from build123d import *

# Parameters (mm, degrees)
CROQUIS1_W              = 42.4
CROQUIS1_H              = 30.8
CROQUIS1_W_2            = 32
CROQUIS1_H_2            = 26.8
SALIENTE_EXTRUIR1_DEPTH = 6
SALIENTE_EXTRUIR2_DEPTH = 14.4
SALIENTE_EXTRUIR3_START = 2
CROQUIS1_4_W            = 42.4
CROQUIS1_4_H            = 30.8
CROQUIS1_4_W_2          = 32
CROQUIS1_4_H_2          = 26.8
CROQUIS1_4_W_3          = 2.2
CROQUIS1_4_H_3          = 2.2
SALIENTE_EXTRUIR3_DEPTH = 2
CORTAR_EXTRUIR1_REACH   = 49.353


with BuildPart() as part:
    # Croquis1 → Saliente-Extruir1 (new body)
    with BuildSketch(Plane(origin=(0, 0, 0), x_dir=(1, 0, 0), z_dir=(0, 1, 0))):
        Rectangle(CROQUIS1_W, CROQUIS1_H)
        Rectangle(CROQUIS1_W_2, CROQUIS1_H_2, mode=Mode.SUBTRACT)
    extrude(amount=-SALIENTE_EXTRUIR1_DEPTH)

    # Croquis1<3> → Saliente-Extruir2 (add)
    with BuildSketch(Plane(origin=(0, 0, 0), x_dir=(1, 0, 0), z_dir=(0, 1, 0))):
        with BuildLine():
            Line((-16, 13.4), (-16, 8.2))
            ThreePointArc((-16, 8.2), (-12.323044738, 9.723044738), (-10.8, 13.4))
            Line((-10.8, 13.4), (-16, 13.4))
        make_face()
        with BuildLine():
            Line((-16, -8.2), (-16, -13.4))
            Line((-16, -13.4), (-10.8, -13.4))
            ThreePointArc((-10.8, -13.4), (-12.323044738, -9.723044738), (-16, -8.2))
        make_face()
        with BuildLine():
            ThreePointArc((10.8, 13.4), (12.323044738, 9.723044738), (16, 8.2))
            Line((16, 8.2), (16, 13.4))
            Line((16, 13.4), (10.8, 13.4))
        make_face()
        with BuildLine():
            ThreePointArc((16, -8.2), (12.323044738, -9.723044738), (10.8, -13.4))
            Line((10.8, -13.4), (16, -13.4))
            Line((16, -13.4), (16, -8.2))
        make_face()
    extrude(amount=-SALIENTE_EXTRUIR2_DEPTH)

    # Croquis1<4> → Saliente-Extruir3 (add)
    # profile 1 of 6: a face of its own
    with BuildSketch(Plane(origin=(0, 0, 0), x_dir=(1, 0, 0), z_dir=(0, 1, 0)).offset(SALIENTE_EXTRUIR3_START)):
        Rectangle(CROQUIS1_4_W, CROQUIS1_4_H)
        Rectangle(CROQUIS1_4_W_2, CROQUIS1_4_H_2, mode=Mode.SUBTRACT)
    # profile 2 of 6: a face of its own
    with BuildSketch(Plane(origin=(0, 0, 0), x_dir=(1, 0, 0), z_dir=(0, 1, 0)).offset(SALIENTE_EXTRUIR3_START)):
        with BuildLine():
            Line((-16, -8.2), (-16, -13.4))
            Line((-16, -13.4), (-10.8, -13.4))
            ThreePointArc((-10.8, -13.4), (-12.323044738, -9.723044738), (-16, -8.2))
        make_face()
    # profile 3 of 6: a face of its own
    with BuildSketch(Plane(origin=(0, 0, 0), x_dir=(1, 0, 0), z_dir=(0, 1, 0)).offset(SALIENTE_EXTRUIR3_START)):
        with BuildLine():
            ThreePointArc((16, -8.2), (12.323044738, -9.723044738), (10.8, -13.4))
            Line((10.8, -13.4), (16, -13.4))
            Line((16, -13.4), (16, -8.2))
        make_face()
    # profile 4 of 6: a face of its own
    with BuildSketch(Plane(origin=(0, 0, 0), x_dir=(1, 0, 0), z_dir=(0, 1, 0)).offset(SALIENTE_EXTRUIR3_START)):
        with BuildLine():
            ThreePointArc((10.8, 13.4), (12.323044738, 9.723044738), (16, 8.2))
            Line((16, 8.2), (16, 13.4))
            Line((16, 13.4), (10.8, 13.4))
        make_face()
    # profile 5 of 6: a face of its own
    with BuildSketch(Plane(origin=(0, 0, 0), x_dir=(1, 0, 0), z_dir=(0, 1, 0)).offset(SALIENTE_EXTRUIR3_START)):
        with BuildLine():
            Line((-16, 13.4), (-16, 8.2))
            ThreePointArc((-16, 8.2), (-12.323044738, 9.723044738), (-10.8, 13.4))
            Line((-10.8, 13.4), (-16, 13.4))
        make_face()
    # profile 6 of 6: a face of its own
    with BuildSketch(Plane(origin=(0, 0, 0), x_dir=(1, 0, 0), z_dir=(0, 1, 0)).offset(SALIENTE_EXTRUIR3_START)):
        with BuildLine():
            ThreePointArc((-16, -8.2), (-12.323044738, -9.723044738), (-10.8, -13.4))
            Line((-10.8, -13.4), (10.8, -13.4))
            ThreePointArc((10.8, -13.4), (12.323044738, -9.723044738), (16, -8.2))
            Line((16, -8.2), (16, 8.2))
            ThreePointArc((16, 8.2), (12.323044738, 9.723044738), (10.8, 13.4))
            Line((10.8, 13.4), (3.2, 13.4))
            Line((3.2, 13.4), (3.2, 11.2))
            Line((3.2, 11.2), (1, 11.2))
            Line((1, 11.2), (1, 13.4))
            Line((1, 13.4), (-1, 13.4))
            Line((-1, 13.4), (-1, 11.2))
            Line((-1, 11.2), (-3.2, 11.2))
            Line((-3.2, 11.2), (-3.2, 13.4))
            Line((-3.2, 13.4), (-10.8, 13.4))
            ThreePointArc((-10.8, 13.4), (-12.323044738, 9.723044738), (-16, 8.2))
            Line((-16, 8.2), (-16, -8.2))
        make_face()
        with Locations((-2.1, 8.1)):
            Rectangle(CROQUIS1_4_W_3, CROQUIS1_4_H_3, mode=Mode.SUBTRACT)
        with Locations((2.1, 8.1)):
            Rectangle(CROQUIS1_4_W_3, CROQUIS1_4_H_3, mode=Mode.SUBTRACT)
    extrude(amount=-SALIENTE_EXTRUIR3_DEPTH)

    # Cortar-Extruir1: up to this face of the body (flat: up to its plane)
    cortar_extruir1_end = Plane(part.part.faces().sort_by_distance((-21.2, -2, 0))[0])
    # Croquis2 → Cortar-Extruir1 (cut, up to the picked face)
    with BuildSketch(Plane(origin=(21.2, 0, 0), x_dir=(0, 0, -1), z_dir=(1, 0, 0)), mode=Mode.PRIVATE) as cortar_extruir1_sk1:
        with BuildLine():
            Line((-2.6, -6), (2.6, -6))
            ThreePointArc((2.6, -6), (0, -3.4), (-2.6, -6))
        make_face()
    cortar_extruir1_tool1 = split(extrude(cortar_extruir1_sk1.sketch, amount=-CORTAR_EXTRUIR1_REACH, mode=Mode.PRIVATE), bisect_by=cortar_extruir1_end, keep=Keep.BOTH, mode=Mode.PRIVATE)
    add(cortar_extruir1_tool1.solids().sort_by(Axis((21.2, -4.896526, 0), (-1, 0, 0)))[0], mode=Mode.SUBTRACT)


solid = part.part
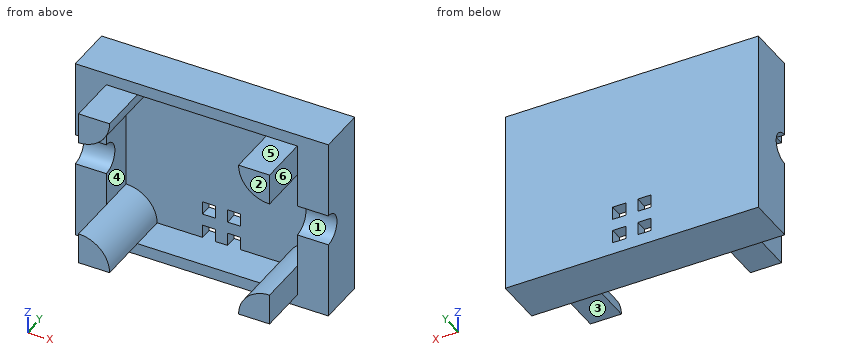
Work out the finished part from the listing and answer in its coordinate system (mm). Face numbers are marked on the shaded views. A direction names the side the tool comes from. Give positions to 0.01 mm unless a question says otherwise; leave off trailing zeros. Order: outer loops, then holes, each group sorted by start corner. A loop starts at its lowest first (then second) coordinate and runs counter-clockwise, first axis right, second up. Notation, with made-up numbers: (9.25, -7) -> (13.25, -7) arc R27 ccw to (13.25, 27) -> close; hole circle Ø5 at (9.5, -12.5). An arc over 180 degrees is marked (long way). Answer as a JSON object with one key per item and string values. Group by question number.
1. Section C-C on y = -12 is taken. Determine the outline of the cut face in (x, z).
2. The mould has two halves that part along Z. Classify the marked faces 1, 2 and 3: released by +Z, released by -Z, zero draft, split by the parting line, or undercut.
3. Consider line 1 along Z through (x, y) = (-1, -2.25); line 2 along X through (y, z) = (-5, 5.5); line 3 along Y through (x, z) = (6, 10). Determine where each line is inside the solid, lowest interval first. Write a range as [from, to].
4. Section A-A on z = -7.5 is taken. Determine the outline of the cut face in (x, y).
5. A tool of negligible diameter and unlimited length cuts with its end or side. For the marked faces 4, 5 and 6, from which of +Z, -Z, +X, -X, +Y, -Y can it reach the whole face along a straight path? Write none if from no direction.
6. Section B-B on x = 7 is taken. Determine the outline of the cut face in (y, z).
7. Flat-ended cylindrical pins translate along their axes: pin 1 Ø10 at (x, z) = (-15.5, 1) entering from -Y; pin 2 Ø1.6 at (x, y) = (-14.5, -12.5) entering from -Z; pin 3 Ø4 at (y, z) = (-9, 2.5) entering from -X; pin 4 Ø6 at (x, z) = (-8, 8.5) entering from -Y. Find the tip coordinate at first contact, or state that the pin passes through.
8. Section D-D on z = 0 is taken. Determine the outline of the cut face in (x, y).
Result sheet:
{
 "1": {"outline": "(-16, -13.4) -> (-10.8, -13.4) arc R5.2 ccw to (-16, -8.2) -> close; (-16, 8.2) arc R5.2 ccw to (-10.8, 13.4) -> (-16, 13.4) -> close; (10.8, -13.4) -> (16, -13.4) -> (16, -8.2) arc R5.2 ccw to start; (10.8, 13.4) arc R5.2 ccw to (16, 8.2) -> (16, 13.4) -> close"},
 "2": {"face 1": "undercut", "face 2": "zero draft", "face 3": "released by -Z"},
 "3": {"line 1": "z = [-15.4, -13.4], [13.4, 15.4]", "line 2": "x = [-21.2, -16], [16, 21.2]", "line 3": "y = [0, 2]"},
 "4": {"outline": "(-21.2, -6) -> (-16, -6) -> (-16, 0) -> (-3.2, 0) -> (-3.2, 2) -> (-21.2, 2) -> close; (-1, 0) -> (1, 0) -> (1, 2) -> (-1, 2) -> close; (3.2, 0) -> (16, 0) -> (16, -6) -> (21.2, -6) -> (21.2, 2) -> (3.2, 2) -> close"},
 "5": {"face 4": "-Y", "face 5": "+Z, +X, -X, -Y", "face 6": "+Z, -Z, +X, -Y"},
 "6": {"outline": "(-6, -15.4) -> (2, -15.4) -> (2, 15.4) -> (-6, 15.4) -> (-6, 13.4) -> (0, 13.4) -> (0, -13.4) -> (-6, -13.4) -> close"},
 "7": {"pin 1": "stops at y = -6", "pin 2": "stops at z = -13.4", "pin 3": "passes through", "pin 4": "stops at y = 0"},
 "8": {"outline": "(-21.2, -3.4) -> (-16, -3.4) -> (-16, 0) -> (16, 0) -> (16, -3.4) -> (21.2, -3.4) -> (21.2, 2) -> (-21.2, 2) -> close"}
}
